```python
from build123d import *

# Parameters (mm, degrees)
FASE1_SIZE  = 6
FASE1_SIZE2 = 3.464101615


with BuildPart() as part:
    # Skizze1 → Rotation1 (revolve)
    with BuildSketch(Plane(origin=(0, 0, 0), x_dir=(0, 0, -1), z_dir=(1, 0, 0))):
        Polygon((115, 0), (115, 25), (95, 25), (95, 20), (90, 15), (-115, 15), (-115, 0), align=None)
    revolve(axis=Axis((0, 0, -115), (0, 0, 1)))

    # Fase1
    fase1_edges = [part.edges().sort_by_distance(p)[0] for p in [
        (0, -25, -95),
    ]]
    fase1_side = [part.faces().sort_by_distance(p)[0] for p in [
        (0, -25, -105),
    ]]
    chamfer(fase1_edges, length=FASE1_SIZE, length2=FASE1_SIZE2, reference=fase1_side[0])

    # Skizze3 → Schnitt-Rotation1 (revolve, cut)
    with BuildSketch(Plane(origin=(0, 0, 115), x_dir=(1, 0, 0), z_dir=(0, -1, 0))):
        Polygon((0, -2.20043031), (0.5, -1.9), (0.5, -0.969948452), (1.06, 0), (0, 0), align=None)
    revolve(axis=Axis((0, 0, 115), (0, 0, -1)), mode=Mode.SUBTRACT)


solid = part.part
```
Source: CAD feature listing. Evaluate the final solid. Frame: model axes, mm. A direction names the side the tool comes from. Round coordinates to 2 decimals unless told otherwise and drop trailing zeros. Loops run counter-clockwise (first coordinate to the right, second up) from the corner with the lowest first, then second, coordinate; pieces in that order, holes last.
1. Access query for faces 1 (the flat face through (14.3, 14.3, -95)), 2 (the flat face through (0, 0, -115)). Directions: +Z, -Z, +X, -X, +Y, -Y. A direction counts if a zero-diameter tool reaches every point of the face in a straight line with its end or side. Return the directions, or none.
2. Section query A-A on z = 76. Output: boundary loops of the cut face in (x, y), and give its area (3 significant figures).
3. Contact query for flat-ended pins moving along their axis: pin 1 (2 mm diameter, centred on x = 17.5, z = 73, fed in from +Y); pin 2 (8 mm diameter, centred on y = -0.5, z = -69, fed in from -X); pin 3 (4 mm diameter, centred on x = -15.5, y = -6.5, fed in from +Z); pin 4 (5 mm diameter, centred on x = -5, z = -50.5, fed in from +Y). Output: stop coordinate, or through.
4. Ray query, L1, parallel to Y at x = 0, z = 113.35; L2, parallel to Z at x = 6, y = -20. Return the intervals inside material, ascending.
Answers below:
1. face 1: +Z
1. face 2: -Z, +X, -X, +Y, -Y
2. outline: circle Ø30 at (0, 0)
2. area: 707 mm2
3. pin 1: passes through
3. pin 2: stops at x = -15
3. pin 3: stops at z = 115
3. pin 4: stops at y = 14.79
4. L1: y = -15 to -0.5, 0.5 to 15
4. L2: z = -115 to -95
